```python
from build123d import *

# Parameters (mm, degrees)
PAD_DEPTH       = 0.245
POCKET_DEPTH    = 0.05
SKETCH004_R     = 0.75
PAD001_DEPTH    = 10.08525
SKETCH005_R     = 3
HOLE_DEPTH      = 26
SKETCH006_R     = 0.495763
POCKET001_DEPTH = 9.580987
SKETCH007_W     = 15
SKETCH007_H     = 15
POCKET002_DEPTH = 5


with BuildPart() as part:
    # Sketch → Pad (new body, symmetric)
    with BuildSketch(Plane.XY):
        with BuildLine():
            Line((0, 0.375), (19.21, 0.375))
            ThreePointArc((19.21, -0.375), (19.585, 0), (19.21, 0.375))
            Line((19.21, -0.375), (0, -0.375))
            ThreePointArc((0, 0.375), (-0.375, 0), (0, -0.375))
        make_face()
    extrude(amount=PAD_DEPTH, both=True)

    # Sketch001 → Revolution (revolve)
    with BuildSketch(Plane.XY):
        with BuildLine():
            Line((0, 0.625), (0, 0))
            Line((0, 0), (0, -0.625))
            ThreePointArc((0, 0.625), (-0.625, 0), (0, -0.625))
        make_face()
    revolve(axis=Axis((0, 0, 0), (0, -1, 0)))

    # Sketch002 → Revolution001 (revolve)
    with BuildSketch(Plane.XY):
        with BuildLine():
            ThreePointArc((19.21, -0.625), (19.835, 0), (19.21, 0.625))
            Line((19.21, 0.625), (19.21, 0))
            Line((19.21, 0), (19.21, -0.625))
        make_face()
    revolve(axis=Axis((19.21, 0, 0), (0, -1, 0)))

    # Sketch003 (on DatumPlane) → Pocket (cut)
    with BuildSketch(Plane.XY.offset(0.25)):
        Polygon((1.05425, -0.16238), (1.148, 0), (1.05425, 0.16238), (0.86675, 0.16238), (0.773, 0), (0.86675, -0.16238), align=None)
    extrude(amount=-POCKET_DEPTH, mode=Mode.SUBTRACT)

    # Sketch004 (on DatumPlane) → Pad001 (join)
    with BuildSketch(Plane.YZ.offset(11.526)):
        Circle(SKETCH004_R)
    extrude(amount=-PAD001_DEPTH)

    # Sketch005 (on DatumPlane) → Hole (cut)
    with BuildSketch(Plane.YZ.offset(11.526)):
        Circle(SKETCH005_R)
    extrude(amount=HOLE_DEPTH, mode=Mode.SUBTRACT)

    # Sketch006 (on DatumPlane) → Pocket001 (cut)
    with BuildSketch(Plane.YZ.offset(11.526)):
        Circle(SKETCH006_R)
    extrude(amount=-POCKET001_DEPTH, mode=Mode.SUBTRACT)

    # Sketch007 (on DatumPlane) → Pocket002 (cut)
    with BuildSketch(Plane.YZ.offset(3.3932)):
        Rectangle(SKETCH007_W, SKETCH007_H)
    extrude(amount=-POCKET002_DEPTH, mode=Mode.SUBTRACT)


solid = part.part
```
Input: part model. Units: mm. Frame: model coordinates. Coordinates: 2 decimals unless noted, no trailing zeros. Write each loop counter-clockwise with the first axis right and the second up, starting at its lowest first coordinate (ties: lowest second). Pieces come first, ordered by that corner, then holes. Notation, with made-up numbers: (69, 23) - (115, 23) arc R26 cw to (115, 61) - close; hole circle Ø10 at (11.5, 20). An arc over 180 degrees is marked (long way). Put each result on its own line as item: value. Start each with the question number.
1) Cut plane C-C (x = 6). Return the cut outline in (y, z), plus the area to 3 significant figures.
2) Mould query, pull axis Z, two halves, no side actions, for faces 1 (the face through (7.52, -0.75, 0.03)), 2 (the face through (7.517, -0.107, -0.484)). Classes: pulls with the +Z half, pulls with the -Z half, needs draft (parallel to the pull), parting line crosses it, or undercut.
3) Cut plane A-A (y = 0). Return the cut outline in (x, z).
4) Ray query, L1, parallel to Z at x = 6.75, y = -0.05; L2, parallel to Y at x = 7.25, z = 0.25. Return the intervals inside material, ascending.
Resolved:
1. outline: circle Ø1.5 at (0, 0); hole circle Ø0.99 at (0, 0)
1. area: 0.995 mm2
2. face 1: parting line crosses it
2. face 2: undercut
3. outline: (3.39, -0.75) - (11.53, -0.75) - (11.53, -0.5) - (3.39, -0.5) - close; (3.39, 0.5) - (11.53, 0.5) - (11.53, 0.75) - (3.39, 0.75) - close
4. L1: z = -0.75 to -0.49, 0.49 to 0.75
4. L2: y = -0.71 to -0.43, 0.43 to 0.71
